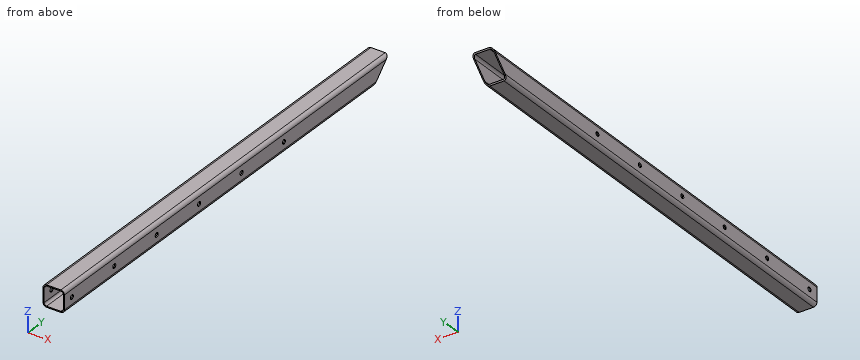
from build123d import *

# Parameters (mm, degrees)
F1_DEPTH = 650
F3_DEPTH = 30.001
F4_R     = 3
F5_DEPTH = 30.001


with BuildPart() as f1:
    # F0 (on Front) → F1 (new body)
    with BuildSketch(Plane.XZ):
        with BuildLine():
            Line((-10, -15), (10, -15))
            ThreePointArc((10, -15), (13.535534, -13.535534), (15, -10))
            Line((15, -10), (15, 10))
            ThreePointArc((15, 10), (13.535534, 13.535534), (10, 15))
            Line((10, 15), (-10, 15))
            ThreePointArc((-10, 15), (-13.535534, 13.535534), (-15, 10))
            Line((-15, 10), (-15, -10))
            ThreePointArc((-15, -10), (-13.535534, -13.535534), (-10, -15))
        make_face()
        with BuildLine():
            ThreePointArc((-10, -13.5), (-12.474874, -12.474874), (-13.5, -10))
            Line((-13.5, -10), (-13.5, 10))
            ThreePointArc((-13.5, 10), (-12.474874, 12.474874), (-10, 13.5))
            Line((-10, 13.5), (10, 13.5))
            ThreePointArc((10, 13.5), (12.474874, 12.474874), (13.5, 10))
            Line((13.5, 10), (13.5, -10))
            ThreePointArc((13.5, -10), (12.474874, -12.474874), (10, -13.5))
            Line((10, -13.5), (-10, -13.5))
        make_face(mode=Mode.SUBTRACT)
    extrude(amount=F1_DEPTH)

    # F2 (on face) → F3 (cut, through all)
    with BuildSketch(Plane.YZ.offset(15)):
        Polygon((0, -15), (0, 15), (-30, -15), align=None)
    extrude(amount=-F3_DEPTH, mode=Mode.SUBTRACT)

    # F4 (on face) → F5 (cut, through all)
    with BuildSketch(Plane.YZ.offset(15)):
        with Locations((-635, 0)):
            Circle(F4_R)
        with Locations((-550, 0)):
            Circle(F4_R)
        with Locations((-465, 0)):
            Circle(F4_R)
        with Locations((-380, 0)):
            Circle(F4_R)
        with Locations((-295, 0)):
            Circle(F4_R)
        with Locations((-210, 0)):
            Circle(F4_R)
    extrude(amount=-F5_DEPTH, mode=Mode.SUBTRACT)


solid = f1.part
Work out the finished part from the listing and answer in its coordinate system (mm). Give positions to 0.01 mm unless a question says otherwise; leave off trailing zeros. Loops run counter-clockwise (first coordinate to the right, second up) from the corner with the lowest first, then second, coordinate; pieces in that order, holes last. Notation, with made-up numbers: (68, 9) -> (75, 9) arc R25 ccw to (75, 35) -> close; hole circle Ø11 at (-14.75, 22.25). An arc over 180 degrees is marked (long way). Use a Markdown table: item, result. Add a question column.
1. Section B-B on y = -67 is taken. Determine the outline of the cut face in (x, z), and give its area (3 significant figures).
2. A flat-ended cylindrical pin translates along its axis: pin 1 Ø10 at (x, z) = (-0.5, -7) entering from -Y. Find the tip coordinate at first contact, or state that the pin passes through.
3. Find the intervals of material crossed by probe 1 along X at (y, z) = (-275.5, -10); probe 2 along Z at (x, y) = (-14.6, -380), in increasing order.
4. Section A-A on x = -4 is taken. Determine the outline of the cut face in (y, z).
Results below:
| question | item | result |
|---|---|---|
| 1 | outline | (-15, -10) arc R5 ccw to (-10, -15) -> (10, -15) arc R5 ccw to (15, -10) -> (15, 10) arc R5 ccw to (10, 15) -> (-10, 15) arc R5 ccw to (-15, 10) -> close; hole (-13.5, -10) arc R3.5 ccw to (-10, -13.5) -> (10, -13.5) arc R3.5 ccw to (13.5, -10) -> (13.5, 10) arc R3.5 ccw to (10, 13.5) -> (-10, 13.5) arc R3.5 ccw to (-13.5, 10) -> close |
| 1 | area | 160 mm^2 |
| 2 | pin 1 | passes through |
| 3 | probe 1 | x = -15 to -13.5, 13.5 to 15 |
| 3 | probe 2 | z = -11.96 to -3, 3 to 11.96 |
| 4 | outline | (-650, -15) -> (-30, -15) -> (-28.5, -13.5) -> (-650, -13.5) -> close; (-650, 13.5) -> (-1.5, 13.5) -> (0, 15) -> (-650, 15) -> close |
